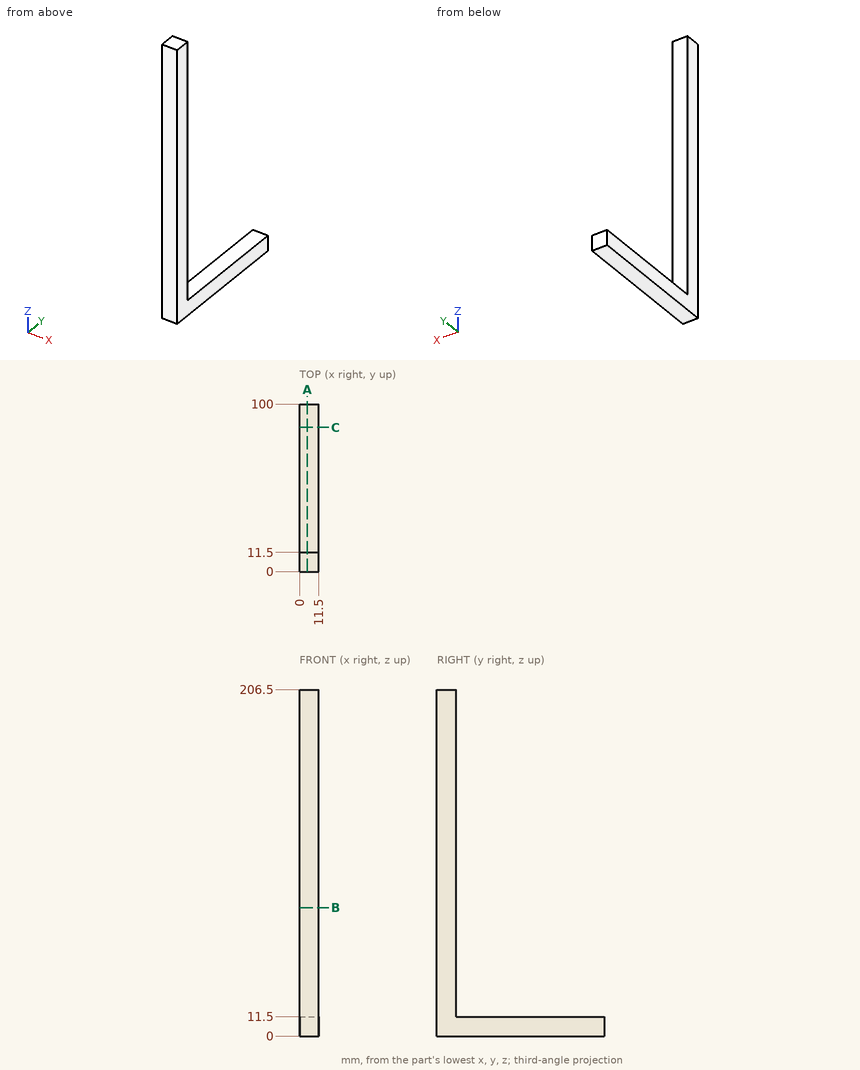
Input: dimensioned drawing with shaded views. Units: mm. Origin: part minimum x, y, z. Coordinates: 2 decimals unless noted, no trailing zeros. Loops run counter-clockwise (first coordinate to the right, second up) from the corner with the lowest first, then second, coordinate; pieces in that order, holes last. Notation, with made-up numbers: M 29.5,31 L 53.5,31 A27 ccw 53.5,55 Z; hole C -15.5,-3.5 d8. An arc over 180 degrees is marked long. Put each result on its own line as item: value.
(1) Cut plane A-A on x = 4.75. Return the cut outline in (y, z).
Answer sheet:
outline: M 0,0 L 100,0 L 100,11.5 L 11.5,11.5 L 11.5,206.5 L 0,206.5 Z
(2) Material intervals for probe 1 along Y at (x, z) = (7.5, 169), sorted ascending.
Answer sheet:
probe 1: y = 0 to 11.5
(3) First-contact query: pin 1 (3.5 mm diameter, centred on x = 4, z = 83, fed in from +Y). Flat tip, straight axial feed; report the tip coordinate or a pass-through.
Answer sheet:
pin 1: stops at y = 11.5
(4) Cut plane B-B on z = 76.5. Return the cut outline in (x, y), then the cut area to 3 significant figures.
Answer sheet:
outline: M 0,0 L 11.5,0 L 11.5,11.5 L 0,11.5 Z
area: 132 mm^2
